Can you work these out from the model? Positions are in its coordinate system, mm. Face numbers are marked on the shaded views. A direction names the side the tool comes from. Round coordinates to 2 decimals unless told otherwise and drop trailing zeros. Loops run counter-clockwise (first coordinate to the right, second up) from the corner with the lowest first, then second, coordinate; pieces in that order, holes last. Notation, with made-up numbers: (-22.5, 29) -> (33.5, 29) arc R30 cw to (33.5, 60) -> close; hole circle Ø9 at (28.5, -15). An arc over 180 degrees is marked (long way). Write item = value, one per line.
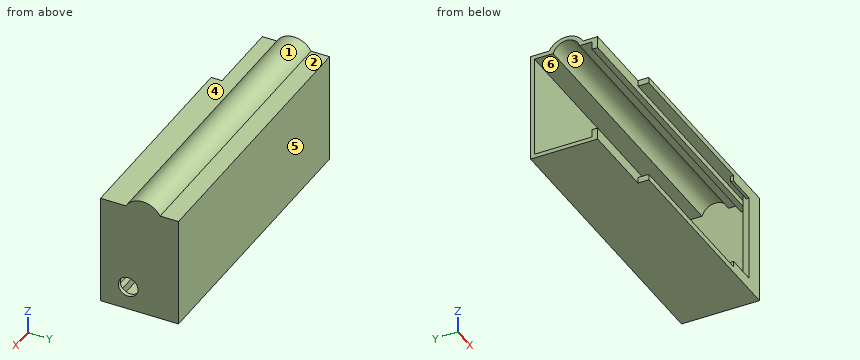
from build123d import *

# Parameters (mm, degrees)
BOSS_EXTRUDE1_DEPTH     = 144
SKETCH2_W               = 4
SKETCH2_H               = 29.171572875
CUT_EXTRUDE1_DEPTH      = 152.921854912
BOSS_EXTRUDE2_DEPTH     = 144
CUT_EXTRUDE2_DEPTH      = 153.922365925
CUT_EXTRUDE2_DEPTH_BACK = 153.922365925
CUT_EXTRUDE3_DEPTH      = 162.298636076
CUT_EXTRUDE3_DEPTH_BACK = 162.298636076
SKETCH6_W               = 39
SKETCH6_H               = 5.5
BOSS_EXTRUDE3_DEPTH     = 56
BOSS_EXTRUDE5_START     = 3
BOSS_EXTRUDE5_DEPTH     = 3
CUT_EXTRUDE5_DEPTH      = 1
CUT_EXTRUDE6_DEPTH      = 155.807138078
CUT_EXTRUDE6_DEPTH_BACK = 155.807138078
SKETCH16_R              = 5
SKETCH17_W              = 82
SKETCH17_H              = 50
CUT_EXTRUDE7_DEPTH      = 3


with BuildPart() as part:
    # Sketch1 → Boss-Extrude1 (new body)
    with BuildSketch(Plane(origin=(0, 0, 0), x_dir=(0, 0, -1), z_dir=(1, 0, 0))):
        Polygon((0, 39.5), (28, 39.5), (28, 0), (22, 0), (22, 1.5), (25, 1.5), (25, 5.5), (22, 5.5), (22, 37.5), (0, 37.5), align=None)
    boss_extrude1 = extrude(amount=BOSS_EXTRUDE1_DEPTH)

    # Mirror1: Boss-Extrude1 across plane
    add(boss_extrude1.mirror(Plane.XY))

    # Sketch2 → Cut-Extrude1 (cut, symmetric)
    with BuildSketch(Plane(origin=(144, 0, 0), x_dir=(0, 0, -1), z_dir=(1, 0, 0))):
        with Locations((24, 22.914213563)):
            Rectangle(SKETCH2_W, SKETCH2_H)
    cut_extrude1 = extrude(amount=CUT_EXTRUDE1_DEPTH, both=True, mode=Mode.SUBTRACT)

    # Mirror2: Cut-Extrude1 across plane
    add(cut_extrude1.mirror(Plane.XY), mode=Mode.SUBTRACT)

    # Sketch3 → Boss-Extrude2 (add)
    with BuildSketch(Plane(origin=(144, 0, 0), x_dir=(0, 0, -1), z_dir=(1, 0, 0))):
        with BuildLine():
            Line((-28, 30.160254038), (-28, 12.839745962))
            ThreePointArc((-28, 12.839745962), (-33, 21.5), (-28, 30.160254038))
        make_face()
    extrude(amount=-BOSS_EXTRUDE2_DEPTH)

    # Sketch4 → Cut-Extrude2 (cut, two sides: drawn at the far end of the back side and taken through both)
    with BuildSketch(Plane(origin=(144, 0, 0), x_dir=(0, 0, -1), z_dir=(1, 0, 0)).offset(-CUT_EXTRUDE2_DEPTH_BACK)):
        with BuildLine():
            Line((-26, 28.036631057), (-26, 14.620223192))
            ThreePointArc((-26, 14.620223192), (-31, 21.328427125), (-26, 28.036631057))
        make_face()
    extrude(amount=CUT_EXTRUDE2_DEPTH + CUT_EXTRUDE2_DEPTH_BACK, mode=Mode.SUBTRACT)

    # Sketch6 → Cut-Extrude3 (cut, two sides: drawn at the far end of the back side and taken through both)
    with BuildSketch(Plane(origin=(0, 0, -28), x_dir=(-1, 0, 0), z_dir=(0, 0, -1)).offset(-CUT_EXTRUDE3_DEPTH_BACK)):
        with Locations((-19.5, 2.75)):
            Rectangle(SKETCH6_W, SKETCH6_H)
    extrude(amount=CUT_EXTRUDE3_DEPTH + CUT_EXTRUDE3_DEPTH_BACK, mode=Mode.SUBTRACT)

    # Sketch7 → Boss-Extrude3 (add)
    with BuildSketch(Plane(origin=(0, 0, -28), x_dir=(-1, 0, 0), z_dir=(0, 0, -1))):
        Polygon((-144, 39.5), (-146, 39.5), (-146, 0), (-136, 0), (-136, 2.997720077), (-144, 2.997720077), align=None)
    extrude(amount=-BOSS_EXTRUDE3_DEPTH)

    # Sketch10 → Boss-Extrude5 (add)
    with BuildSketch(Plane(origin=(144, 0, 0), x_dir=(0, 0, -1), z_dir=(1, 0, 0)).offset(BOSS_EXTRUDE5_START)):
        with BuildLine():
            Line((-28, 30.160254038), (-28, 12.839745962))
            ThreePointArc((-28, 12.839745962), (-33, 21.5), (-28, 30.160254038))
        make_face()
    extrude(amount=-BOSS_EXTRUDE5_DEPTH)

    # Sketch15 → Cut-Extrude5 (cut)
    with BuildSketch(Plane(origin=(147, 0, 0), x_dir=(0, 0, -1), z_dir=(1, 0, 0))):
        with BuildLine():
            Line((-28, 12.839745962), (-28, 30.160254038))
            ThreePointArc((-28, 30.160254038), (-33, 21.5), (-28, 12.839745962))
        make_face()
    extrude(amount=-CUT_EXTRUDE5_DEPTH, mode=Mode.SUBTRACT)

    # Sketch16 → Cut-Extrude6 (cut, two sides: drawn at the far end of the back side and taken through both)
    with BuildSketch(Plane(origin=(146, 0, 0), x_dir=(0, 0, -1), z_dir=(1, 0, 0)).offset(-CUT_EXTRUDE6_DEPTH_BACK)):
        with Locations((16, 14)):
            Circle(SKETCH16_R)
    extrude(amount=CUT_EXTRUDE6_DEPTH + CUT_EXTRUDE6_DEPTH_BACK, mode=Mode.SUBTRACT)

    # Sketch17 → Cut-Extrude7 (cut)
    with BuildSketch(Plane.XZ):
        with Locations((80, 0)):
            Rectangle(SKETCH17_W, SKETCH17_H)
    extrude(amount=-CUT_EXTRUDE7_DEPTH, mode=Mode.SUBTRACT)


solid = part.part
1. Suppose I cut it at B-B, the plane x = 32. List the corners of the cut face in (y, z) for me, and give its area (3 significant figures).
Entries:
outline = (5.5, -28) -> (39.5, -28) -> (39.5, 28) -> (30.16, 28) arc R10 ccw to (12.84, 28) -> (5.5, 28) -> (5.5, 22) -> (8.33, 22) -> (8.33, 26) -> (14.62, 26) arc R7 cw to (28.04, 26) -> (37.5, 26) -> (37.5, -26) -> (8.33, -26) -> (8.33, -22) -> (5.5, -22) -> close
area = 275 mm²
2. Suppose I cut it at D-D, the plane z = 19.5. List the corners of the cut face in (x, y) for me, and give its area (3 significant figures).
Entries:
outline = (0, 37.5) -> (144, 37.5) -> (144, 3) -> (136, 3) -> (136, 0) -> (146, 0) -> (146, 39.5) -> (0, 39.5) -> close
area = 391 mm²
3. We'd pull the mould along Z, two halves only. Please class the marked faces 4, 5 and 6: released by +Z, released by -Z, zero draft, split by the parting line, or undercut.
Entries:
face_4 = released by +Z
face_5 = zero draft
face_6 = undercut
4. I'm going to push flat-ended pins straight in: pin 1 (8 mm diameter, centred on x = 16.5, y = 5, fed in from +Z); pin 2 (12 mm diameter, centred on y = 16, z = 0, fed in from -X); pin 3 (2.5 mm diameter, centred on y = 2, z = 7.5, fed in from -X). Where does each tip first touch, or does it pass through?
Entries:
pin_1 = 28
pin_2 = 144
pin_3 = 136
5. I need wall thicknesses on line 1 (Y direction, x = 145, z = -16); line 2 (Y direction, x = 80.5, z = 23); line 3 (Z direction, x = 67, y = 31). Which ranges of each line are inside material? Lowest first, please. Write a range as [from, to].
Entries:
line_1 = [0, 9], [19, 39.5]
line_2 = [5.5, 8.33], [37.5, 39.5]
line_3 = [-28, -26], [26, 28]
6. For the marked faces 1, 2 and 3, which set-ups out of +Z, -Z, +X, -X, +Y, -Y let a thin tool reach every point of the face, with its end or its side?
Entries:
face_1 = +Z, +X, -X
face_2 = +Z, +X, -X, +Y
face_3 = -X
7. Suppose I cut it at C-C, the plane y = 35. List the corners of the cut face in (x, z) for me.
Entries:
outline = (0, -28) -> (146, -28) -> (146, 28) -> (0, 28) -> (0, 26) -> (144, 26) -> (144, -26) -> (0, -26) -> close
8. Suppose I cut it at A-A, the plane z = -16. List the corners of the cut face in (x, y) for me.
Entries:
outline = (0, 37.5) -> (144, 37.5) -> (144, 19) -> (146, 19) -> (146, 39.5) -> (0, 39.5) -> close; (136, 0) -> (146, 0) -> (146, 9) -> (144, 9) -> (144, 3) -> (136, 3) -> close
